Can you work these out from the model? Positions are in its coordinate system, mm. Face numbers are marked on the shaded views. A direction names the side the tool comes from. Coordinates: 2 decimals unless noted, no trailing zeros. Order: outer loops, then holes, each group sorted by start corner. A loop starts at its lowest first (then second) coordinate and runs counter-clockwise, first axis right, second up. Notation, with made-up numbers: (53, 4.5) -> (88, 4.5) arc R27 cw to (88, 22.5) -> close; hole circle Ø8 at (-22, -21). An arc over 180 degrees is marked (long way). Use a Markdown table: item, result. Add a question column.
1. We'd pull the mould along X, two halves only. Please class the marked faces 1, 2 and 3: pulls with the +X half, pulls with the -X half, needs draft (parallel to the pull), parting line crosses it, or undercut.
2. For pin 1 Ø7 at (y, z) = (18, -3) entering from +X; pin 2 Ø12 at (y, z) = (8.5, 21.5) entering from -X; pin 3 Ø12 at (y, z) = (20, -34.5) entering from +X; pin 4 Ø4 at (x, z) = (-20, -14.5) entering from -Y, each with a flat end and sliding along its axis, tell me the tip position at first contact or that it passes through.
3. Suppose I cut it at B-B, the plane z = 0. List the corners of the cut face in (x, y) for me, then the cut area to 3 significant figures.
4. Suppose I cut it at D-D, the plane y = 4.5. List the corners of the cut face in (x, z) for me.
5. Suppose I cut it at C-C, the plane y = 26.5. List the corners of the cut face in (x, z) for me.
6. If I drill on line 1 along Z through (x, y) = (31.5, 7); line 2 along Z through (x, y) = (38, 18.75); line 3 along Z through (x, y) = (29.5, 7), over which ranges is the centre line in solid material (lowest first)? Write a range as from..to.
7. Suppose I cut it at A-A, the plane x = 0. List the corners of the cut face in (y, z) for me.
8. For the marked faces 4 and 5, which set-ups out of +Z, -Z, +X, -X, +Y, -Y let a thin tool reach every point of the face, with its end or its side?
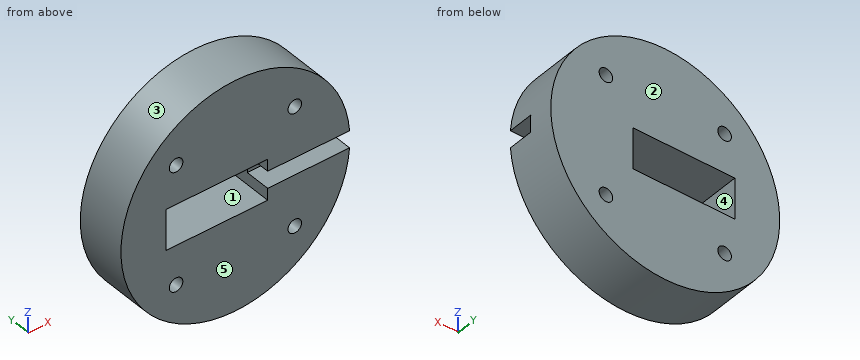
```python
from build123d import *

# Parameters (mm, degrees)
SKETCH_1_R          = 67.5
EXTRUDE_1_DEPTH     = 30
SKETCH_2_W          = 60
SKETCH_2_H          = 24
CUT_EXTRUDE_1_DEPTH = 101.062480481
SKETCH_3_W          = 10
SKETCH_3_H          = 15
CUT_EXTRUDE_2_DEPTH = 97
SKETCH_4_R          = 4
CUT_EXTRUDE_3_DEPTH = 101.062480481


with BuildPart() as part:
    # 草图1 → 凸台-拉伸1 (new body)
    with BuildSketch(Plane(origin=(0, 0, 0), x_dir=(1, 0, 0), z_dir=(0, 1, 0))):
        with Locations(Location((0, 0, 0), (0, 0, 270))):
            Circle(SKETCH_1_R)
    extrude(amount=EXTRUDE_1_DEPTH)

    # 草图2 → 切除-拉伸1 (cut, through all)
    with BuildSketch(Plane(origin=(0, 30, 0), x_dir=(1, 0, 0), z_dir=(0, 1, 0))):
        with Locations((-11, 0)):
            Rectangle(SKETCH_2_W, SKETCH_2_H)
    extrude(amount=-CUT_EXTRUDE_1_DEPTH, mode=Mode.SUBTRACT)

    # 草图3 → 切除-拉伸2 (cut)
    with BuildSketch(Plane(origin=(0, 0, 0), x_dir=(0, 0, -1), z_dir=(1, 0, 0))):
        with Locations((0, 7.5)):
            Rectangle(SKETCH_3_W, SKETCH_3_H)
    extrude(amount=CUT_EXTRUDE_2_DEPTH, mode=Mode.SUBTRACT)

    # 草图4 → 切除-拉伸3 (cut, through all)
    with BuildSketch(Plane(origin=(0, 30, 0), x_dir=(1, 0, 0), z_dir=(0, 1, 0))):
        with Locations(Location((35.001785669, 35.001785669, 0), (0, 0, 270))):
            Circle(SKETCH_4_R)
        with Locations(Location((35.001785669, -35.001785669, 0), (0, 0, 270))):
            Circle(SKETCH_4_R)
        with Locations(Location((-35.001785669, -35.001785669, 0), (0, 0, 270))):
            Circle(SKETCH_4_R)
        with Locations(Location((-35.001785669, 35.001785669, 0), (0, 0, 270))):
            Circle(SKETCH_4_R)
    extrude(amount=-CUT_EXTRUDE_3_DEPTH, mode=Mode.SUBTRACT)


solid = part.part
```
Worked out:
| question | item | result |
|---|---|---|
| 1 | face 1 | undercut |
| 1 | face 2 | needs draft |
| 1 | face 3 | parting line crosses it |
| 2 | pin 1 | stops at x = 67.5 |
| 2 | pin 2 | stops at x = -65.7 |
| 2 | pin 3 | stops at x = 61.19 |
| 2 | pin 4 | stops at y = 0 |
| 3 | outline | (-67.5, 0) -> (-41, 0) -> (-41, 30) -> (-67.5, 30) -> close; (19, 15) -> (67.5, 15) -> (67.5, 30) -> (19, 30) -> close |
| 3 | area | 1,520 mm² |
| 4 | outline | (-41, -12) -> (-41, 12) -> (19, 12) -> (19, 5) -> (67.31, 5) arc R67.5 ccw (long way) to (67.31, -5) -> (19, -5) -> (19, -12) -> close; hole circle Ø8 at (-35, -35); hole circle Ø8 at (-35, 35); hole circle Ø8 at (35, -35); hole circle Ø8 at (35, 35) |
| 5 | outline | circle Ø135 at (0, 0); hole (-41, -12) -> (19, -12) -> (19, 12) -> (-41, 12) -> close; hole circle Ø8 at (-35, -35); hole circle Ø8 at (-35, 35); hole circle Ø8 at (35, -35); hole circle Ø8 at (35, 35) |
| 6 | line 1 | z = -59.7..-36.94, -33.07..-5, 5..33.07, 36.94..59.7 |
| 6 | line 2 | z = -55.79..-37.65, -32.35..32.35, 37.65..55.79 |
| 6 | line 3 | z = -60.71..-5, 5..60.71 |
| 7 | outline | (0, -67.5) -> (30, -67.5) -> (30, -12) -> (0, -12) -> close; (0, 12) -> (30, 12) -> (30, 67.5) -> (0, 67.5) -> close |
| 8 | face 4 | +Y, -Y |
| 8 | face 5 | +Z, -Z, +X, -X, -Y |
